Part print with two shaded views. Sizes in mm from the minimum x, y, z corner. A direction names the side the tool comes from. Round coordinates to 2 decimals unless told otherwise and drop trailing zeros. Order: outer loops, then holes, each group sorted by start corner. A loop starts at its lowest first (then second) coordinate and runs counter-clockwise, first axis right, second up. Notation, with made-up numbers: M 14,-29 L 37,-29 A25 cw 37,2 Z; hole C 22.25,7.5 d10. An arc over 180 degrees is marked long. Put each result on its own line as item: value.
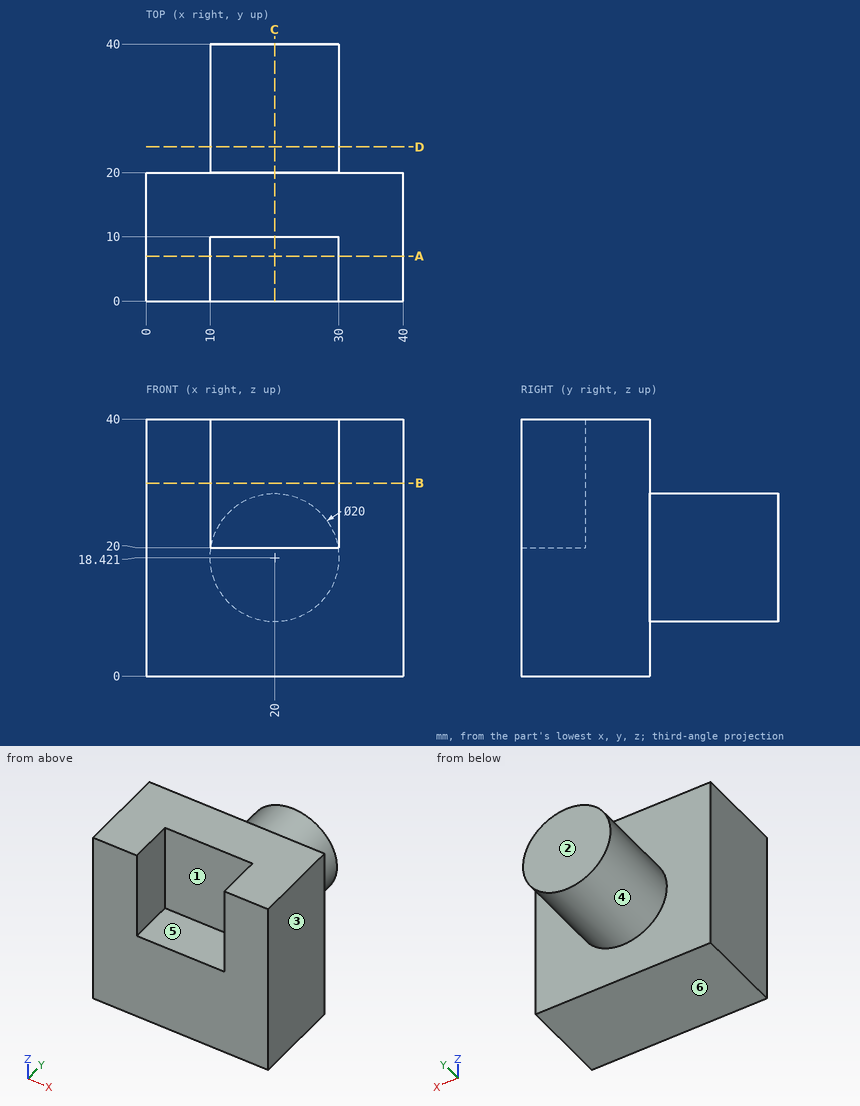
Item 1: Probe line 1 along Y through (x, z) = (21, 22); line 2 along Y through (x, z) = (12.5, 4). List the from-to ranges inside material, lowest first. Write a range as [from, to].
Answers below:
line 1: [10, 40]
line 2: [0, 20]
Item 2: Mould opens along X. For the marked faces 1, 2 and 3 say: pulls with the +X half, pulls with the -X half, needs draft (parallel to the pull), parting line crosses it, or undercut.
Answers below:
face 1: undercut
face 2: needs draft
face 3: pulls with the +X half
Item 3: Band-saw the part on D-D on y = 24. Give the cut face in (x, z).
Answers below:
outline: C 20,18.42 d20
Item 4: Tool access for the marked faces 4, 5 and 6: list every direction of +Z, -Z, +X, -X, +Y, -Y with a clear straight run to the whole face (end or side of a thin tool).
Answers below:
face 4: +Y
face 5: +Z, -Y
face 6: -Z, +X, -X, +Y, -Y
Item 5: Pin check, flat tips, straight feed: P1, Ø5, axis at x = 24.5, y = 5, coming from the +Z side; P2, Ø8, axis at x = 10, z = 33.5, coming from the +Y side; P3, Ø5, axis at y = 25, z = 11.5, coming from the -X side. Stop position of each tip, or through.
Answers below:
P1: z = 20
P2: y = 20
P3: x = 11.03
Item 6: Band-saw the part on A-A on y = 7. Give the cut face in (x, z).
Answers below:
outline: M 0,0 L 40,0 L 40,40 L 30,40 L 30,20 L 10,20 L 10,40 L 0,40 Z
Item 7: Band-saw the part on C-C on x = 20. Give the cut face in (y, z).
Answers below:
outline: M 0,0 L 20,0 L 20,8.42 L 40,8.42 L 40,28.42 L 20,28.42 L 20,40 L 10,40 L 10,20 L 0,20 Z
Item 8: Band-saw the part on B-B on z = 30. Give the cut face in (x, y), and give its area (3 significant figures).
Answers below:
outline: M 0,0 L 10,0 L 10,10 L 30,10 L 30,0 L 40,0 L 40,20 L 0,20 Z
area: 600 mm²
